```python
from build123d import *

# Parameters (mm, degrees)
ESQUISSE1_W             = 20.2
ESQUISSE1_H             = 20
ESQUISSE1_W_2           = 37.8
ESQUISSE1_H_2           = 16
BOSS_EXTRU_1_DEPTH      = 42.5
ESQUISSE2_R             = 12
ENL_V_MAT_EXTRU_1_DEPTH = 25
D_GAGEMENT_M31_D        = 3.2
D_GAGEMENT_M32_D        = 3.2
D_GAGEMENT_M33_D        = 3.2
ENL_V_MAT_EXTRU_2_REACH = 32.2
ESQUISSE11_W            = 15
ESQUISSE11_H            = 6


with BuildPart() as part:
    # Esquisse1 → Boss.-Extru.1 (new body)
    with BuildSketch(Plane.XY):
        Polygon((0, 0), (72, 0), (72, -24), (28, -24), (28, -30), (24, -30), (24, -24), (12, -24), (12, -30), (8, -30), (8, -24), (0, -24), (0, -18), (6, -18), (6, -6), (0, -6), align=None)
        with Locations((18.1, -12)):
            Rectangle(ESQUISSE1_W, ESQUISSE1_H, mode=Mode.SUBTRACT)
        with Locations((49.1, -12)):
            Rectangle(ESQUISSE1_W_2, ESQUISSE1_H_2, mode=Mode.SUBTRACT)
    extrude(amount=BOSS_EXTRU_1_DEPTH)

    # Esquisse2 → Enlèv. mat.-Extru.1 (cut, through all)
    with BuildSketch(Plane.XZ.offset(24)):
        with Locations((50, 21.25)):
            Circle(ESQUISSE2_R)
    extrude(amount=-ENL_V_MAT_EXTRU_1_DEPTH, mode=Mode.SUBTRACT)

    # Dégagement M31 (through all)
    with Locations(Plane(origin=(0, -24, 0), x_dir=(-1, 0, 0), z_dir=(0, -1, 0))):
        with Locations((-50, -21.25), (-34.5, -5.75), (-65.5, -36.75), (-65.5, -5.75), (-34.5, -36.75)):
            Hole(D_GAGEMENT_M31_D / 2)

    # Dégagement M32 (through all)
    with Locations(Plane(origin=(28, 0, 0), x_dir=(0, 0, -1), z_dir=(1, 0, 0))):
        with Locations((-10, -27), (-32.5, -27)):
            Hole(D_GAGEMENT_M32_D / 2)

    # Dégagement M33 (through all)
    with Locations(Plane(origin=(0, -24, 0), x_dir=(-1, 0, 0), z_dir=(0, -1, 0))):
        with Locations((-3, -10), (-3, -32.5)):
            Hole(D_GAGEMENT_M33_D / 2)

    # Esquisse11 → Enlèv. mat.-Extru.2 (cut, up to next)
    with BuildSketch(Plane(origin=(30.2, 0, 0), x_dir=(0, 0, -1), z_dir=(1, 0, 0)), mode=Mode.PRIVATE) as enl_v_mat_extru_2_sk1:
        with Locations((-7.5, -12)):
            Rectangle(ESQUISSE11_W, ESQUISSE11_H)
    enl_v_mat_extru_2_tool1 = extrude(enl_v_mat_extru_2_sk1.sketch, amount=-ENL_V_MAT_EXTRU_2_REACH, mode=Mode.PRIVATE) & part.part
    add(enl_v_mat_extru_2_tool1.solids().sort_by_distance((30.2, -12, 7.5))[0], mode=Mode.SUBTRACT)
    # Esquisse11 → Enlèv. mat.-Extru.2 (cut, up to next)
    with BuildSketch(Plane(origin=(30.2, 0, 0), x_dir=(0, 0, -1), z_dir=(1, 0, 0)), mode=Mode.PRIVATE) as enl_v_mat_extru_2_sk2:
        with Locations((-35, -12)):
            Rectangle(ESQUISSE11_W, ESQUISSE11_H)
    enl_v_mat_extru_2_tool2 = extrude(enl_v_mat_extru_2_sk2.sketch, amount=-ENL_V_MAT_EXTRU_2_REACH, mode=Mode.PRIVATE) & part.part
    add(enl_v_mat_extru_2_tool2.solids().sort_by_distance((30.2, -12, 35))[0], mode=Mode.SUBTRACT)


solid = part.part
```
The model under review builds one solid part; all positions refer to its coordinate system, in mm. A direction names the side the tool comes from. Give positions to 0.01 mm unless a question says otherwise; leave off trailing zeros. Write each loop counter-clockwise with the first axis right and the second up, starting at its lowest first coordinate (ties: lowest second). Pieces come first, ordered by that corner, then holes.
(1) Consider section D-D, the plane x = 34.5. Give the boundary of the cut face in (y, z).
(2) Consider section B-B, the plane x = 15. Give the boundary of the cut face in (y, z), and give its area (3 significant figures).
(3) Tool access review of faces 4 (the flat face through (29, -12, 15)), 5 (the flat face through (29, -15, 35)), 6 (the flat face through (18, -2, 21)): name each direction out of +Z, -Z, +X, -X, +Y, -Y from which nothing blocks a thin tool from reaching the whole face with its end or side.
(4) To check wall thickness, follow L1, parallel to X at y = -18.5, z = 6; L2, parallel to X at y = -12.75, z = 22.5; L3, parallel to X at y = -21.55, z = 36.75. State the ranges of each line that lie inside material, in increasing order.
(5) For P1, Ø8, axis at y = -10.5, z = 23, coming from the -X side; P2, Ø5, axis at y = -27, z = 18.5, coming from the +X side; P3, Ø3, axis at y = -27, z = 21, coming from the -X side, all flat-tipped, find the tip position at first contact; note any pin that passes through.
(6) The part is to be moulded in two halves that separate along X. For faces 1 (the flat face through (3, -6, 21)), 2 (the flat face through (8, -27, 21)), 3 (the flat face through (36, -20, 21)), say which applies: released by +X, released by -X, zero draft, split by the parting line, or undercut.
(7) Consider section C-C, the plane y = -27. Give the boundary of the cut face in (x, z), and give its area (3 significant figures).
(8) Consider section A-A, the plane y = -3. Give the number of separate pieces and of enclosed holes in the cut face, and give its area (3 significant figures).
Returned:
1. outline: (-24, 0) - (-20, 0) - (-20, 4.15) - (-24, 4.15) - close; (-24, 7.35) - (-20, 7.35) - (-20, 35.15) - (-24, 35.15) - close; (-24, 38.35) - (-20, 38.35) - (-20, 42.5) - (-24, 42.5) - close; (-4, 0) - (0, 0) - (0, 4.15) - (-4, 4.15) - close; (-4, 7.35) - (0, 7.35) - (0, 35.15) - (-4, 35.15) - close; (-4, 38.35) - (0, 38.35) - (0, 42.5) - (-4, 42.5) - close
2. outline: (-24, 0) - (-22, 0) - (-22, 42.5) - (-24, 42.5) - close; (-2, 0) - (0, 0) - (0, 42.5) - (-2, 42.5) - close
2. area: 170 mm2
3. face 4: -Z
3. face 5: +Z
3. face 6: +Z, -Z
4. L1: x = 0 to 8, 28.2 to 30.2, 68 to 72
4. L2: x = 6 to 8, 28.2 to 30.2, 68 to 72
4. L3: x = 0 to 8, 28.2 to 32.9, 36.1 to 63.9, 67.1 to 72
5. P1: stops at x = 6
5. P2: stops at x = 28
5. P3: stops at x = 8
6. face 1: zero draft
6. face 2: released by -X
6. face 3: undercut
7. outline: (8, 0) - (12, 0) - (12, 8.4) - (8, 8.4) - close; (8, 11.6) - (12, 11.6) - (12, 30.9) - (8, 30.9) - close; (8, 34.1) - (12, 34.1) - (12, 42.5) - (8, 42.5) - close; (24, 0) - (28, 0) - (28, 8.4) - (24, 8.4) - close; (24, 11.6) - (28, 11.6) - (28, 30.9) - (24, 30.9) - close; (24, 34.1) - (28, 34.1) - (28, 42.5) - (24, 42.5) - close
7. area: 289 mm2
8. separate pieces: 2
8. enclosed holes: 7
8. area: 1,700 mm2
